Work out the finished part from the listing and answer in its coordinate system (mm). Round coordinates to 2 decimals unless told otherwise and drop trailing zeros. Loops run counter-clockwise (first coordinate to the right, second up) from the corner with the lowest first, then second, coordinate; pieces in that order, holes last. Notation, with made-up numbers: (25.5, -12.5) - (58.5, -12.5) arc R26 ccw to (58.5, 5.5) - close; hole circle Ø6 at (15, 22). An arc over 180 degrees is marked (long way). Return JSON: item names as keys, results as strings.
from build123d import *

# Parameters (mm, degrees)
SKETCH1_W           = 10
SKETCH1_H           = 10
SKETCH1_R           = 3.5
BOSS_EXTRUDE1_DEPTH = 60
SKETCH2_R           = 3.5
BOSS_EXTRUDE2_DEPTH = 40


with BuildPart() as part:
    # Sketch1 → Boss-Extrude1 (new body)
    with BuildSketch(Plane(origin=(0, 0, 0), x_dir=(1, 0, 0), z_dir=(0, 1, 0))):
        Rectangle(SKETCH1_W, SKETCH1_H)
        with Locations(Location((0, 0, 0), (0, 0, 270))):
            Circle(SKETCH1_R, mode=Mode.SUBTRACT)
    extrude(amount=BOSS_EXTRUDE1_DEPTH)

    # Sketch2 → Boss-Extrude2 (add)
    with BuildSketch(Plane(origin=(0, 0, 0), x_dir=(1, 0, 0), z_dir=(0, 1, 0))):
        with Locations(Location((0, 0, 0), (0, 0, 270))):
            Circle(SKETCH2_R)
    extrude(amount=BOSS_EXTRUDE2_DEPTH)


solid = part.part
1) Find the intervals of material crossed by L1, parallel to X at y = 54, z = 0; L2, parallel to Y at x = -1.5, z = -1; L3, parallel to X at y = 44.5, z = -2.5, in increasing order.
Verdict:
{"L1": "x = -5 to -3.5, 3.5 to 5", "L2": "y = 0 to 40", "L3": "x = -5 to -2.45, 2.45 to 5"}
2) Determine the mould class of faces 1 (the cylindrical face through (-3.417, 49.86, -0.759)), 2 (the flat face through (-2.3, 60, -3.4)), 3 (the flat face through (-5, 30, 0)), 4 (the flat face through (0, 40, 0)) for opening direction X: pulls with the +X half, pulls with the -X half, needs draft (parallel to the pull), parting line crosses it, or undercut.
Verdict:
{"face 1": "undercut", "face 2": "needs draft", "face 3": "pulls with the -X half", "face 4": "undercut"}
3) Section A-A (z = 0) is taken. Give the vertices of the cut face in (x, y), and give its area (3 significant figures).
Verdict:
{"outline": "(-5, 0) - (5, 0) - (5, 60) - (3.5, 60) - (3.5, 40) - (-3.5, 40) - (-3.5, 60) - (-5, 60) - close", "area": "460 mm2"}
4) A flat-ended cylindrical pin translates along its axis: pin 1 (1 mm diameter, centred on x = 2.5, z = -1, fed in from +Y). Find the tip coordinate at first contact, or state that the pin passes through.
Verdict:
{"pin 1": "stops at y = 40"}
5) Section C-C (x = 2) is taken. Give the vertices of the cut face in (y, z), and give its area (3 significant figures).
Verdict:
{"outline": "(0, -5) - (60, -5) - (60, -2.87) - (40, -2.87) - (40, 2.87) - (60, 2.87) - (60, 5) - (0, 5) - close", "area": "485 mm2"}
6) Section B-B (y = 49) is taken. Give the vertices of the cut face in (x, z).
Verdict:
{"outline": "(-5, -5) - (5, -5) - (5, 5) - (-5, 5) - close; hole circle Ø7 at (0, 0)"}
